Autodesk Inventor part; units mm, degrees
ref_plane "YZ Plane" through (0, 0, 0) normal (1, 0, 0) x (0, 1, 0)
ref_plane "XZ Plane" through (0, 0, 0) normal (0, 1, 0) x (-1, 0, 0)
ref_plane "XY Plane" through (0, 0, 0) normal (0, 0, 1) x (1, 0, 0)
sketch "スケッチ1" plane through (0, 0, 0) normal (0, 0, 1) x (1, 0, 0)
  circle A0 centre (0, 0) radius 1.5
  dimension "d0" = 3
extrude "押し出し1" add sketch "スケッチ1" along normal blind 12
sketch "スケッチ2" plane through (0, 0, 12) normal (0, 0, 1) x (1, 0, 0)
  circle A0 centre (0, 0) radius 3.45
  dimension "d3" = 6.9
extrude "押し出し2" add sketch "スケッチ2" along normal blind 1.9
fillet "フィレット1" radius 1.9 1 edges at (-3.45, 0, 13.9)
thread "ねじ1"
properties part number "M3トラス頭ネジ　12" material "鉄 灰色"
Geometry check sheet. Reference: the model listing, model coordinates, mm. A direction names the side the tool comes from. Round coordinates to 2 decimals unless told otherwise and drop trailing zeros. Write each loop counter-clockwise with the first axis right and the second up, starting at its lowest first coordinate (ties: lowest second). Pieces come first, ordered by that corner, then holes. Notation, with made-up numbers: (-20, 34.5) - (-4, 34.5) arc R28 cw to (-4, 65.5) - close; hole circle Ø10 at (-15.75, 65). An arc over 180 degrees is marked (long way). Write each question's results on one line, items separated by ' | '.
(1) Sectioned sample at A-A, the plane z = 7.5. Enter the section's corners in (x, y), plus the area to 3 significant figures.
Computed:
outline: circle Ø3 at (0, 0) | area: 7.07 mm^2
(2) Set-up check for faces 1 (the face through (0, 0, 13.9)), 2 (the face through (1.5, -0.7, 12)): record each of +Z, -Z, +X, -X, +Y, -Y from which the full face is reachable in a straight line by a thin tool's end or side.
Computed:
face 1: +Z, +X, -X, +Y, -Y | face 2: -Z
(3) Thickness scan on probe 1 along X at (y, z) = (1.25, 4.75); probe 2 along Z at (x, y) = (-1, -3); probe 3 along Z at (x, y) = (-2.75, -1.75). Record the ranges inside material, lowest first. Write a range as from..to.
Computed:
probe 1: x = -0.83..0.83 | probe 2: z = 12..13.01 | probe 3: z = 12..12.83
(4) Depth check by flat-ended pin: pin 1 Ø1 at (y, z) = (1.5, 2.5) entering from +X; pin 2 Ø1.5 at (x, y) = (-2, 2.5) entering from -Z; pin 3 Ø4 at (x, z) = (2, 9) entering from +Y; pin 4 Ø1.5 at (x, z) = (0.5, 11.5) entering from +Y. Enter the tip coordinate at first touch or a pass-through.
Computed:
pin 1: stops at x = 1.12 | pin 2: stops at z = 12 | pin 3: stops at y = 1.5 | pin 4: stops at y = 3.45
